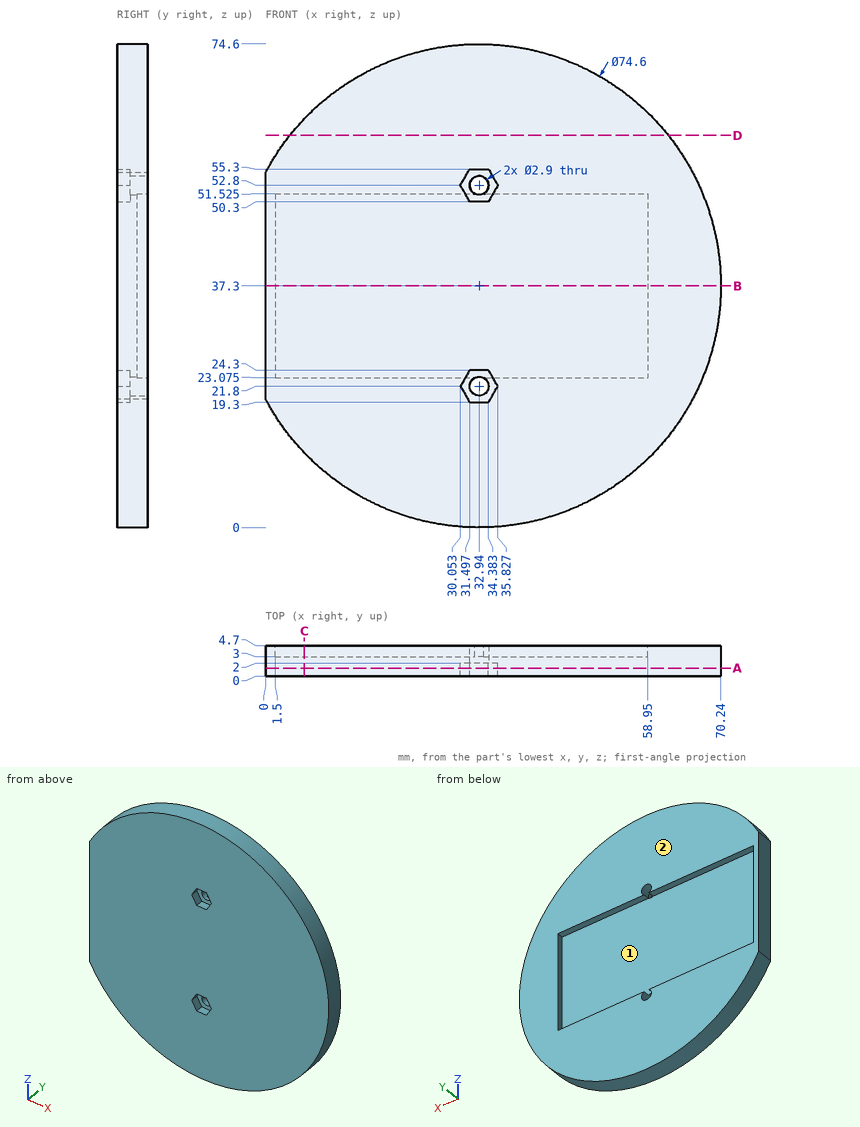
Here's the drawing with two shaded views (mm, measured from the low corner). I have some questions. Coordinates: 2 decimals unless noted, no trailing zeros. Loops run counter-clockwise (first coordinate to the right, second up) from the corner with the lowest first, then second, coordinate; pieces in that order, holes last. Notation, with made-up numbers: (81.25, 15.25) - (123.25, 15.25) arc R25 ccw to (123.25, 51.25) - close; hole circle Ø2 at (32.25, 15.5). An arc over 180 degrees is marked (long way). Answer as CSV lines item,"result". Start each with the question number.
1) Suppose I cut it at A-A (y = 1.2). Please give me the cut outline in (x, z), plus the area to 3 significant figures.
2) Suppose I cut it at C-C (x = 6). Please give me the cut outline in (y, z) (1 decimal).
3) For pin 1 (1.9 mm diameter, centred on x = 24, y = 4, fed in from -Z); pin 2 (1.4 mm diameter, centred on x = 49.5, y = 4, fed in from -Z); pin 3 (10 mm diameter, centred on x = 22.5, z = 30.5, fed in from +Y); pin 4 (2.5 mm diameter, centred on x = 32.94, z = 21.8, fed in from -Y), each with a flat end and sliding along its axis, tell me the tip position at first contact or that it passes through.
4) Thinking about a two-plate mould opening in X: for the marked faces 1 and 2, which applies, pulls with the +X half, pulls with the -X half, needs draft (parallel to the pull), parting line crosses it, or undercut?
5) Suppose I cut it at B-B (z = 37.3). Please give me the cut outline in (x, y).
6) Suppose I cut it at D-D (z = 60.5). Please give me the cut outline in (x, y).
7) I need wall thicknesses on line 1 (Z direction, x = 30.5, y = 0.5) (1 decimal); line 2 (Y direction, x = 8.5, z = 26); line 3 (Z direction, x = 20.5, y = 3.65) (1 decimal). Which ranges of each line are inside material? Lowest first, please. Write a range as from..to.
Check result:
1,outline,"(0, 19.8) arc R37.3 ccw (long way) to (0, 54.8) - close; hole (30.05, 21.8) - (31.5, 19.3) - (34.38, 19.3) - (35.83, 21.8) - (34.38, 24.3) - (31.5, 24.3) - close; hole (30.05, 52.8) - (31.5, 50.3) - (34.38, 50.3) - (35.83, 52.8) - (34.38, 55.3) - (31.5, 55.3) - close"
1,area,"4,220 mm²"
2,outline,"(0, 11.5) - (4.7, 11.5) - (4.7, 23.1) - (3, 23.1) - (3, 51.5) - (4.7, 51.5) - (4.7, 63.1) - (0, 63.1) - close"
3,pin 1,"stops at z = 0.87"
3,pin 2,"stops at z = 3.54"
3,pin 3,"stops at y = 3"
3,pin 4,"passes through"
4,face 1,"undercut"
4,face 2,"needs draft"
5,outline,"(0, 0) - (70.24, 0) - (70.24, 4.7) - (58.95, 4.7) - (58.95, 3) - (1.5, 3) - (1.5, 4.7) - (0, 4.7) - close"
6,outline,"(3.73, 0) - (62.15, 0) - (62.15, 4.7) - (3.73, 4.7) - close"
7,line 1,"z = 0.1..21, 22.6..52, 53.6..74.5"
7,line 2,"y = 0..3"
7,line 3,"z = 2.1..23.1, 51.5..72.5"
